Work out the finished part from the listing and answer in its coordinate system (mm). A direction names the side the tool comes from. Coordinates: 2 decimals unless noted, no trailing zeros. Order: outer loops, then holes, each group sorted by start corner. A loop starts at its lowest first (then second) coordinate and runs counter-clockwise, first axis right, second up. Notation, with made-up numbers: M 52.5,16.5 L 58.5,16.5 A23 cw 58.5,25.5 Z; hole C 56.5,-34.75 d9. An arc over 180 degrees is marked long. Write item = value, one per line. Start each with the question number.
Q1. Find section B-B on z = 1.75. Give the vertices of the cut face in (x, y), and give its area (3 significant figures).
Q2. A tool of negligible diameter and unlimited length cuts with its end or side. For faces 1 (the flat face through (-23, 4, 9)), 2 (the cylindrical face through (-24, 2, 1)), 3 (the flat face through (-1, 2, 9)), 4 (the flat face through (23, 4, 9)), from which of +Z, -Z, +X, -X, +Y, -Y can it reach the whole face along a straight path? Write none if from no direction.
Q3. Find section A-A on z = 15.5. Give the vertices of the cut face in (x, y).
Q4. Each of these flat-tipped pins is pushed along its axis until it touches: P1, Ø1, axis at y = 4, z = 13.5, coming from the -X side; P2, Ø5, axis at x = -23, z = 13.5, coming from the +Y side; P3, Ø1, axis at y = 11.5, z = 5.5, coming from the +X side. Where does it stop, or does it pass through?
Q5. Straight lines are drawn through the part: line 1 along Z through (x, y) = (-13, 13.5); line 2 along Z through (x, y) = (-20, 1); line 3 along Y through (x, z) = (-21, 13.5). For each, find the intervals that lie inside material, in ascending order.
```python
from build123d import *

# Parameters (mm, degrees)
F1_DEPTH = 18
F2_R     = 3.5
F4_R     = 5


with BuildPart() as f1:
    # F0 (on Top) → F1 (new body)
    with BuildSketch(Plane.XY):
        with BuildLine():
            Line((26, 4), (19.595918, 4))
            ThreePointArc((19.595918, 4), (0, 20), (-19.595918, 4))
            Line((-19.595918, 4), (-26, 4))
            Line((-26, 4), (-26, 0))
            Line((-26, 0), (-7, 0))
            Line((-7, 0), (-1.5, 1.5))
            Line((-1.5, 1.5), (0, 3))
            Line((0, 3), (1.5, 1.5))
            Line((1.5, 1.5), (7, 0))
            Line((7, 0), (26, 0))
            Line((26, 0), (26, 4))
        make_face()
    extrude(amount=F1_DEPTH)

    # F2 (on face) → F3 (revolve, cut)
    with BuildSketch(Plane.XZ):
        with Locations((19, 9)):
            Circle(F2_R)
    revolve(axis=Axis((0, 0, 6.141683), (0, 0, -1)), mode=Mode.SUBTRACT)

    # F4
    f4_edges = [f1.edges().sort_by_distance(p)[0] for p in [
        (26, 2, 18),
        (26, 2, 0),
        (-26, 2, 0),
        (-26, 2, 18),
    ]]
    fillet(f4_edges, radius=F4_R)


solid = f1.part
```
Findings below:
q1.outline = M -24.8,0 L -7,0 L -1.5,1.5 L 0,3 L 1.5,1.5 L 7,0 L 24.8,0 L 24.8,4 L 19.6,4 A20 ccw -19.6,4 L -24.8,4 Z
q1.area = 653 mm^2
q2.face_1 = +Z, -Z, -X, +Y
q2.face_2 = -Z, -X, +Y, -Y
q2.face_3 = +Z, -Z, -Y
q2.face_4 = +Z, -Z, +X, +Y
q3.outline = M -25.33,0 L -7,0 L -1.5,1.5 L 0,3 L 1.5,1.5 L 7,0 L 25.33,0 L 25.33,4 L 19.6,4 A20 ccw -19.6,4 L -25.33,4 Z
q4.P1 = -26
q4.P2 = 4
q4.P3 = 16.7
q5.line_1 = 0 to 5.51, 12.49 to 18
q5.line_2 = 0 to 5.65, 12.35 to 18
q5.line_3 = 0 to 4
